```python
from build123d import *

# Parameters (mm, degrees)
BOSS_EXTRUDE1_DEPTH     = 500
BOSS_EXTRUDE2_START     = 30
SKETCH2_W               = 500
SKETCH2_H               = 40
BOSS_EXTRUDE2_DEPTH     = 30
RIB1_REACH              = 507.173
SKETCH4_WALL_W          = 1057.782982674
SKETCH4_WALL_H          = 10
LPATTERN1_COUNT         = 10
LPATTERN1_PITCH         = 50
MIRROR1_COPY_1_REACH    = 507.173
MIRROR1_COPY_1_SKETCH_W = 1057.782982674
MIRROR1_COPY_1_SKETCH_H = 10
MIRROR1_COPY_2_REACH    = 507.173
MIRROR1_COPY_2_SKETCH_W = 1057.782982674
MIRROR1_COPY_2_SKETCH_H = 10
MIRROR1_COPY_3_REACH    = 507.173
MIRROR1_COPY_3_SKETCH_W = 1057.782982674
MIRROR1_COPY_3_SKETCH_H = 10
MIRROR1_COPY_4_REACH    = 507.173
MIRROR1_COPY_4_SKETCH_W = 1057.782982674
MIRROR1_COPY_4_SKETCH_H = 10
MIRROR1_COPY_5_REACH    = 507.173
MIRROR1_COPY_5_SKETCH_W = 1057.782982674
MIRROR1_COPY_5_SKETCH_H = 10
MIRROR1_COPY_6_REACH    = 507.173
MIRROR1_COPY_6_SKETCH_W = 1057.782982674
MIRROR1_COPY_6_SKETCH_H = 10
MIRROR1_COPY_7_REACH    = 507.173
MIRROR1_COPY_7_SKETCH_W = 1057.782982674
MIRROR1_COPY_7_SKETCH_H = 10
MIRROR1_COPY_8_REACH    = 507.173
MIRROR1_COPY_8_SKETCH_W = 1057.782982674
MIRROR1_COPY_8_SKETCH_H = 10
MIRROR1_COPY_9_REACH    = 507.173
MIRROR1_COPY_9_SKETCH_W = 1057.782982674
MIRROR1_COPY_9_SKETCH_H = 10
SKETCH5_W               = 400
SKETCH5_H               = 20.700317686
CUT_EXTRUDE1_DEPTH      = 5


with BuildPart() as part:
    # Sketch1 → Boss-Extrude1 (new body)
    with BuildSketch(Plane.XY):
        with BuildLine():
            ThreePointArc((-5.714285714, 39.589732744), (-9.948716593, 33.926730437), (-4.285714286, 29.692299558))
            ThreePointArc((-4.285714286, 29.692299558), (30, 0), (-4.285714286, -29.692299558))
            ThreePointArc((-4.285714286, -29.692299558), (-9.948716593, -33.926730437), (-5.714285714, -39.589732744))
            ThreePointArc((-5.714285714, -39.589732744), (40, 0), (-5.714285714, 39.589732744))
        make_face()
    extrude(amount=BOSS_EXTRUDE1_DEPTH)

    # Sketch2 → Boss-Extrude2 (add)
    with BuildSketch(Plane(origin=(0, 0, 0), x_dir=(0, 0, -1), z_dir=(1, 0, 0)).offset(BOSS_EXTRUDE2_START)):
        with Locations((-250, 0)):
            Rectangle(SKETCH2_W, SKETCH2_H)
    extrude(amount=BOSS_EXTRUDE2_DEPTH)

    # Sketch4 wall → Rib1 (add, up to next)
    with BuildSketch(Plane(origin=(38.733961597, 27.992162595, 0), x_dir=(-0.936077158958, 0.351794759025, 0), z_dir=(0.351794759025, 0.936077158958, 0)), mode=Mode.PRIVATE) as rib1_sk1:
        with Locations((0, 5)):
            Rectangle(SKETCH4_WALL_W, SKETCH4_WALL_H)
    rib1_tool1 = extrude(rib1_sk1.sketch, amount=-RIB1_REACH, mode=Mode.PRIVATE) - part.part
    rib1 = rib1_tool1.solids().sort_by_distance((38.733961597, 27.992162595, 0))[0]
    add(rib1)

    # LPattern1: Rib1 ×10
    with Locations(*[(0, 0, i * LPATTERN1_PITCH) for i in range(1, LPATTERN1_COUNT)]):
        add(rib1)

    # Mirror1: Rib1 across plane
    add(rib1.mirror(Plane.ZX))

    # Mirror1 copy 1 sketch → Mirror1 copy 1 (add, up to next)
    with BuildSketch(Plane(origin=(38.733961597, -27.992162595, 50), x_dir=(-0.936077158958, -0.351794759025, 0), z_dir=(0.351794759025, -0.936077158958, 0)), mode=Mode.PRIVATE) as mirror1_copy_1_sk1:
        with Locations((0, -5)):
            Rectangle(MIRROR1_COPY_1_SKETCH_W, MIRROR1_COPY_1_SKETCH_H)
    mirror1_copy_1_tool1 = extrude(mirror1_copy_1_sk1.sketch, amount=-MIRROR1_COPY_1_REACH, mode=Mode.PRIVATE) - part.part
    add(mirror1_copy_1_tool1.solids().sort_by_distance((38.733961597, -27.992162595, 50))[0])

    # Mirror1 copy 2 sketch → Mirror1 copy 2 (add, up to next)
    with BuildSketch(Plane(origin=(38.733961597, -27.992162595, 100), x_dir=(-0.936077158958, -0.351794759025, 0), z_dir=(0.351794759025, -0.936077158958, 0)), mode=Mode.PRIVATE) as mirror1_copy_2_sk1:
        with Locations((0, -5)):
            Rectangle(MIRROR1_COPY_2_SKETCH_W, MIRROR1_COPY_2_SKETCH_H)
    mirror1_copy_2_tool1 = extrude(mirror1_copy_2_sk1.sketch, amount=-MIRROR1_COPY_2_REACH, mode=Mode.PRIVATE) - part.part
    add(mirror1_copy_2_tool1.solids().sort_by_distance((38.733961597, -27.992162595, 100))[0])

    # Mirror1 copy 3 sketch → Mirror1 copy 3 (add, up to next)
    with BuildSketch(Plane(origin=(38.733961597, -27.992162595, 150), x_dir=(-0.936077158958, -0.351794759025, 0), z_dir=(0.351794759025, -0.936077158958, 0)), mode=Mode.PRIVATE) as mirror1_copy_3_sk1:
        with Locations((0, -5)):
            Rectangle(MIRROR1_COPY_3_SKETCH_W, MIRROR1_COPY_3_SKETCH_H)
    mirror1_copy_3_tool1 = extrude(mirror1_copy_3_sk1.sketch, amount=-MIRROR1_COPY_3_REACH, mode=Mode.PRIVATE) - part.part
    add(mirror1_copy_3_tool1.solids().sort_by_distance((38.733961597, -27.992162595, 150))[0])

    # Mirror1 copy 4 sketch → Mirror1 copy 4 (add, up to next)
    with BuildSketch(Plane(origin=(38.733961597, -27.992162595, 200), x_dir=(-0.936077158958, -0.351794759025, 0), z_dir=(0.351794759025, -0.936077158958, 0)), mode=Mode.PRIVATE) as mirror1_copy_4_sk1:
        with Locations((0, -5)):
            Rectangle(MIRROR1_COPY_4_SKETCH_W, MIRROR1_COPY_4_SKETCH_H)
    mirror1_copy_4_tool1 = extrude(mirror1_copy_4_sk1.sketch, amount=-MIRROR1_COPY_4_REACH, mode=Mode.PRIVATE) - part.part
    add(mirror1_copy_4_tool1.solids().sort_by_distance((38.733961597, -27.992162595, 200))[0])

    # Mirror1 copy 5 sketch → Mirror1 copy 5 (add, up to next)
    with BuildSketch(Plane(origin=(38.733961597, -27.992162595, 250), x_dir=(-0.936077158958, -0.351794759025, 0), z_dir=(0.351794759025, -0.936077158958, 0)), mode=Mode.PRIVATE) as mirror1_copy_5_sk1:
        with Locations((0, -5)):
            Rectangle(MIRROR1_COPY_5_SKETCH_W, MIRROR1_COPY_5_SKETCH_H)
    mirror1_copy_5_tool1 = extrude(mirror1_copy_5_sk1.sketch, amount=-MIRROR1_COPY_5_REACH, mode=Mode.PRIVATE) - part.part
    add(mirror1_copy_5_tool1.solids().sort_by_distance((38.733961597, -27.992162595, 250))[0])

    # Mirror1 copy 6 sketch → Mirror1 copy 6 (add, up to next)
    with BuildSketch(Plane(origin=(38.733961597, -27.992162595, 300), x_dir=(-0.936077158958, -0.351794759025, 0), z_dir=(0.351794759025, -0.936077158958, 0)), mode=Mode.PRIVATE) as mirror1_copy_6_sk1:
        with Locations((0, -5)):
            Rectangle(MIRROR1_COPY_6_SKETCH_W, MIRROR1_COPY_6_SKETCH_H)
    mirror1_copy_6_tool1 = extrude(mirror1_copy_6_sk1.sketch, amount=-MIRROR1_COPY_6_REACH, mode=Mode.PRIVATE) - part.part
    add(mirror1_copy_6_tool1.solids().sort_by_distance((38.733961597, -27.992162595, 300))[0])

    # Mirror1 copy 7 sketch → Mirror1 copy 7 (add, up to next)
    with BuildSketch(Plane(origin=(38.733961597, -27.992162595, 350), x_dir=(-0.936077158958, -0.351794759025, 0), z_dir=(0.351794759025, -0.936077158958, 0)), mode=Mode.PRIVATE) as mirror1_copy_7_sk1:
        with Locations((0, -5)):
            Rectangle(MIRROR1_COPY_7_SKETCH_W, MIRROR1_COPY_7_SKETCH_H)
    mirror1_copy_7_tool1 = extrude(mirror1_copy_7_sk1.sketch, amount=-MIRROR1_COPY_7_REACH, mode=Mode.PRIVATE) - part.part
    add(mirror1_copy_7_tool1.solids().sort_by_distance((38.733961597, -27.992162595, 350))[0])

    # Mirror1 copy 8 sketch → Mirror1 copy 8 (add, up to next)
    with BuildSketch(Plane(origin=(38.733961597, -27.992162595, 400), x_dir=(-0.936077158958, -0.351794759025, 0), z_dir=(0.351794759025, -0.936077158958, 0)), mode=Mode.PRIVATE) as mirror1_copy_8_sk1:
        with Locations((0, -5)):
            Rectangle(MIRROR1_COPY_8_SKETCH_W, MIRROR1_COPY_8_SKETCH_H)
    mirror1_copy_8_tool1 = extrude(mirror1_copy_8_sk1.sketch, amount=-MIRROR1_COPY_8_REACH, mode=Mode.PRIVATE) - part.part
    add(mirror1_copy_8_tool1.solids().sort_by_distance((38.733961597, -27.992162595, 400))[0])

    # Mirror1 copy 9 sketch → Mirror1 copy 9 (add, up to next)
    with BuildSketch(Plane(origin=(38.733961597, -27.992162595, 450), x_dir=(-0.936077158958, -0.351794759025, 0), z_dir=(0.351794759025, -0.936077158958, 0)), mode=Mode.PRIVATE) as mirror1_copy_9_sk1:
        with Locations((0, -5)):
            Rectangle(MIRROR1_COPY_9_SKETCH_W, MIRROR1_COPY_9_SKETCH_H)
    mirror1_copy_9_tool1 = extrude(mirror1_copy_9_sk1.sketch, amount=-MIRROR1_COPY_9_REACH, mode=Mode.PRIVATE) - part.part
    add(mirror1_copy_9_tool1.solids().sort_by_distance((38.733961597, -27.992162595, 450))[0])

    # Sketch5 → Cut-Extrude1 (cut)
    with BuildSketch(Plane(origin=(60, 0, 0), x_dir=(0, 0, -1), z_dir=(1, 0, 0))):
        with Locations((-250, 0)):
            Rectangle(SKETCH5_W, SKETCH5_H)
    extrude(amount=-CUT_EXTRUDE1_DEPTH, mode=Mode.SUBTRACT)


solid = part.part
```
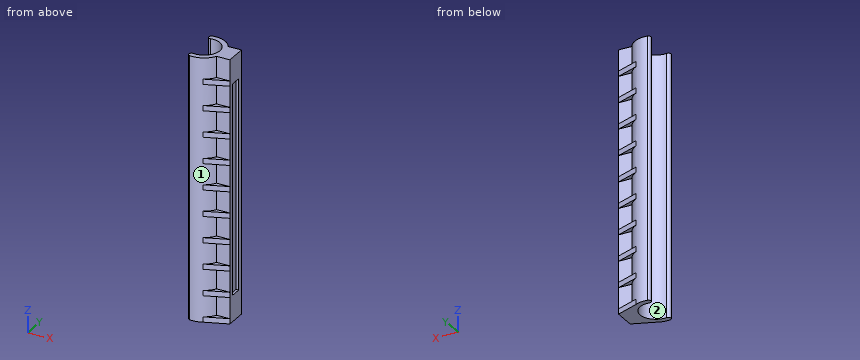
The model under review builds one solid part; all positions refer to its coordinate system, in mm. Face numbers are marked on the shaded views. Give positions to 0.01 mm unless a question says otherwise; leave off trailing zeros. Write each loop counter-clockwise with the first axis right and the second up, starting at its lowest first coordinate (ties: lowest second). Pieces come first, ordered by that corner, then holes. Notation, with made-up numbers: M 56.25,17.5 L 95.25,17.5 A9 cw 95.25,32.5 Z; hole C -35.75,33 d2. An arc over 180 degrees is marked long. Answer in a Markdown table with one row per item.
Item 1: Add section C-C on z = 374. Give the boundary of the cut face in (x, y).
Check sheet entries:
| item | result |
|---|---|
| outline | M -5.71,-39.59 A40 ccw 34.64,-20 L 60,-20 L 60,-10.35 L 55,-10.35 L 55,10.35 L 60,10.35 L 60,20 L 34.64,20 A40 ccw -5.71,39.59 A5 ccw -4.29,29.69 A30 cw long -4.29,-29.69 A5 ccw Z |
Item 2: For line 1 along Y through (x, z) = (1, 62.5); line 2 along X through (y, z) = (4, 325.5); line 3 along X through (y, z) = (0, 115.5), list the stretches that pass through material, from the lowest coordinate up.
Check sheet entries:
| item | result |
|---|---|
| line 1 | -39.99 to -29.98, 29.98 to 39.99 |
| line 2 | 29.73 to 55 |
| line 3 | 30 to 55 |
Item 3: For P1, Ø17.5, axis at x = 40.5, y = -31.5, coming from the +Z side; P2, Ø1.5, axis at x = 40, z = 54, coming from the -Y side; P3, Ø6, axis at y = 12.5, z = 121, coming from the -X side, all flat-tipped, find the tip position at first contact; note any pin that passes through.
Check sheet entries:
| item | result |
|---|---|
| P1 | z = 460 |
| P2 | y = -27.8 |
| P3 | x = 25.69 |
Item 4: Add section A-A on x = 0. Give the boundary of the cut face in (y, z), plus the area to 4 significant figures.
Check sheet entries:
| item | result |
|---|---|
| outline | M -40,0 L -30,0 L -30,500 L -40,500 Z; M 30,0 L 40,0 L 40,500 L 30,500 Z |
| area | 10,000 mm2 |
Item 5: Add section B-B on y = 0. Give the boundary of the cut face in (x, z).
Check sheet entries:
| item | result |
|---|---|
| outline | M 30,0 L 60,0 L 60,50 L 55,50 L 55,450 L 60,450 L 60,500 L 30,500 Z |
Item 6: Draft analysis for pull direction Y (two halves, no side actions). For the marked faces 1 and 2, state which applies: +Y half, -Y half, draft (parallel to the pull), parting line (faces both ways), or undercut.
Check sheet entries:
| item | result |
|---|---|
| face 1 | -Y half |
| face 2 | undercut |
